Can you work these out from the model? Positions are in its coordinate system, mm. A direction names the side the tool comes from. Give positions to 0.01 mm unless a question says otherwise; leave off trailing zeros. Loops run counter-clockwise (first coordinate to the right, second up) from the corner with the lowest first, then second, coordinate; pieces in that order, holes last. Notation, with made-up numbers: (-19, 33) - (34, 33) arc R24 ccw to (34, 53) - close; hole circle Ø2 at (0, 68.5). An arc over 180 degrees is marked (long way). Use a Markdown table: item, result. Add a question column.
```python
from build123d import *

# Parameters (mm, degrees)
BOSS_EXTRUDE1_DEPTH  = 20
CUT_EXTRUDE2_START   = -16.729038
SKETCH3_R            = 3
CUT_EXTRUDE2_DEPTH   = 16.729038
SKETCH2_R            = 9
CUT_EXTRUDE1_DEPTH   = 2
SKETCH5_R            = 1.7
CUT_EXTRUDE3_DEPTH   = 16.729037413
CIRPATTERN1_COUNT    = 4
SKETCH6_R            = 1.7
CUT_EXTRUDE4_DEPTH   = 23.112367583
LPATTERN1_COUNT      = 2
LPATTERN1_PITCH      = 20
LPATTERN1_COUNT_DIR2 = 2
LPATTERN1_PITCH_DIR2 = 35


with BuildPart() as part:
    # Sketch1 → Boss-Extrude1 (new, symmetric)
    with BuildSketch(Plane(origin=(0, 0, 0), x_dir=(0, 0, -1), z_dir=(1, 0, 0))):
        Polygon((0, 0), (34, 0), (34, -16.729037413), (-23.112367583, -16.729037413), (-23.112367583, 75), (0, 75), align=None)
    extrude(amount=BOSS_EXTRUDE1_DEPTH, both=True)

    # Sketch3 → Cut-Extrude2 (cut)
    with BuildSketch(Plane(origin=(0, 0, 0), x_dir=(1, 0, 0), z_dir=(0, 1, 0)).offset(CUT_EXTRUDE2_START)):
        with Locations(Location((0, 17, 0), (0, 0, 270))):
            Circle(SKETCH3_R)
    extrude(amount=CUT_EXTRUDE2_DEPTH, mode=Mode.SUBTRACT)

    # Sketch2 → Cut-Extrude1 (cut)
    with BuildSketch(Plane(origin=(0, 0, 0), x_dir=(1, 0, 0), z_dir=(0, 1, 0))):
        with Locations(Location((0, 17, 0), (0, 0, 270))):
            Circle(SKETCH2_R)
    extrude(amount=-CUT_EXTRUDE1_DEPTH, mode=Mode.SUBTRACT)

    # Sketch5 → Cut-Extrude3 (cut)
    with BuildSketch(Plane(origin=(0, 0, 0), x_dir=(1, 0, 0), z_dir=(0, 1, 0))):
        with Locations(Location((0, 28, 0), (0, 0, 270))):
            Circle(SKETCH5_R)
    cut_extrude3 = extrude(amount=-CUT_EXTRUDE3_DEPTH, mode=Mode.SUBTRACT)

    # CirPattern1: Cut-Extrude3 ×4 about axis
    cirpattern1_axis = Axis((0, 0, -17), (0, 1, 0))
    for i in range(1, CIRPATTERN1_COUNT):
        add(cut_extrude3.rotate(cirpattern1_axis, i * 360 / CIRPATTERN1_COUNT), mode=Mode.SUBTRACT)

    # Sketch6 → Cut-Extrude4 (cut)
    with BuildSketch(Plane(origin=(0, 0, 0), x_dir=(-1, 0, 0), z_dir=(0, 0, -1))):
        with Locations(Location((10, 55, 0), (0, 0, 90))):
            Circle(SKETCH6_R)
    cut_extrude4 = extrude(amount=-CUT_EXTRUDE4_DEPTH, mode=Mode.SUBTRACT)

    # LPattern1: Cut-Extrude4 2 × 2
    with Locations(*[(i * LPATTERN1_PITCH, -j * LPATTERN1_PITCH_DIR2, 0) for i in range(LPATTERN1_COUNT) for j in range(LPATTERN1_COUNT_DIR2) if (i, j) != (0, 0)]):
        add(cut_extrude4, mode=Mode.SUBTRACT)


solid = part.part
```
1. If we mould it in two halves opening along X, with no side actions, what happens to faces 4 (the face through (-10.65, 21.57, 11.39)), 5 (the face through (20, 20, 7)), 6 (the face through (5, 0, -9))? For each: released by +X, released by -X, zero draft, split by the parting line, or undercut.
2. Will these pins go through, and if not, where does the flat tip stop? P1, Ø3, axis at x = 0, z = -6, coming from the +Y side; P2, Ø9, axis at x = 2.5, z = -14.5, coming from the +Y side; P3, Ø5.5, axis at x = 11, z = -17, coming from the +Y side; P4, Ø12, axis at x = -9.5, y = 44.5, coming from the -Z side.
3. Suppose I cut it at A-A (z = -17). List the corners of the cut face in (x, y) for me.
4. Suppose I cut it at B-B (y = 55). List the corners of the cut face in (x, z) for me.
5. Suppose I cut it at D-D (z = -6). List the corners of the cut face in (x, y) for me, and give its area (3 significant figures).
6. Suppose I cut it at C-C (x = 0). List the corners of the cut face in (y, z) for me.
7. Please list where these lines run through material, in increasing order: line 1 along X through (y, z) = (20, 17); line 2 along Y through (x, z) = (-8.5, 3); line 3 along X through (y, z) = (20.5, 16). Write a range as [from, to].
8. On a 3-axis mill with a long thin cutter (end or side, diameter ignored), from which of +Z, -Z, +X, -X, +Y, -Y can I reach the whole of each face in a straight line? I mean faces 1 (the face through (0, 38, 0)), 2 (the face through (0, 28, 23.112)), 3 (the face through (0, -2, -13)). Say none if no direction works.
Results below:
| question | item | result |
|---|---|---|
| 1 | face 4 | undercut |
| 1 | face 5 | released by +X |
| 1 | face 6 | zero draft |
| 2 | P1 | through |
| 2 | P2 | y = -2 |
| 2 | P3 | y = 0 |
| 2 | P4 | z = 0 |
| 3 | outline | (-20, -16.73) - (-12.7, -16.73) - (-12.7, 0) - (-20, 0) - close; (-9.3, -16.73) - (-3, -16.73) - (-3, -2) - (-9, -2) - (-9, 0) - (-9.3, 0) - close; (3, -16.73) - (9.3, -16.73) - (9.3, 0) - (9, 0) - (9, -2) - (3, -2) - close; (12.7, -16.73) - (20, -16.73) - (20, 0) - (12.7, 0) - close |
| 4 | outline | (-20, 0) - (-11.7, 0) - (-11.7, 23.11) - (-20, 23.11) - close; (-8.3, 0) - (8.3, 0) - (8.3, 23.11) - (-8.3, 23.11) - close; (11.7, 0) - (20, 0) - (20, 23.11) - (11.7, 23.11) - close |
| 5 | outline | (-20, -16.73) - (-1.7, -16.73) - (-1.7, 0) - (-20, 0) - close; (1.7, -16.73) - (20, -16.73) - (20, 0) - (1.7, 0) - close |
| 5 | area | 612 mm² |
| 6 | outline | (-16.73, -34) - (0, -34) - (0, -29.7) - (-16.73, -29.7) - close; (-16.73, -26.3) - (0, -26.3) - (0, -26) - (-2, -26) - (-2, -20) - (-16.73, -20) - close; (-16.73, -14) - (-2, -14) - (-2, -8) - (0, -8) - (0, -7.7) - (-16.73, -7.7) - close; (-16.73, -4.3) - (0, -4.3) - (0, 0) - (75, 0) - (75, 23.11) - (-16.73, 23.11) - close |
| 7 | line 1 | [-20, -11.7], [-8.3, 8.3], [11.7, 20] |
| 7 | line 2 | [-16.73, 19.2], [20.8, 54.2], [55.8, 75] |
| 7 | line 3 | [-20, -11.62], [-8.38, 8.38], [11.62, 20] |
| 8 | face 1 | -Z, +X, -X, +Y |
| 8 | face 2 | +Z, +X, -X, +Y, -Y |
| 8 | face 3 | +Y |
